Here's the drawing with two shaded views (mm, measured from the low corner). I have some questions. A direction names the side the tool comes from. Coordinates: 2 decimals unless noted, no trailing zeros. Order: outer loops, then holes, each group sorted by start corner. A loop starts at its lowest first (then second) coordinate and runs counter-clockwise, first axis right, second up. Notation, with made-up numbers: (-4.5, -9.5) -> (18.5, -9.5) arc R18 ccw to (18.5, 21.5) -> close; hole circle Ø7 at (59.5, -12.75). An arc over 180 degrees is marked (long way). Answer in a Markdown table with one row per item. Add a question column.
1. Imagine slicing it at D-D on z = 6. Write out the boundary of the cut face in (x, y).
2. On a 3-axis mill with a long thin cutter (end or side, diameter ignored), from which of +Z, -Z, +X, -X, +Y, -Y can I reach the whole of each face in a straight line? I mean the marked faces 1, 2 and 3. Say none if no direction works.
3. Will these pins go through, and if not, where does the flat tip stop? pin 1 (5 mm diameter, centred on y = 4.5, z = 12.5, fed in from -X); pin 2 (10 mm diameter, centred on y = 11, z = 10.5, fed in from +X).
4. Imagine slicing it at A-A on y = 10. Write out the boundary of the cut face in (x, z), plus the area to 3 significant figures.
5. Imagine slicing it at B-B on z = 22. Write out the boundary of the cut face in (x, y).
6. If I drill on line 1 along X through (y, z) = (3.5, 27.25); line 2 along Z through (x, y) = (2.5, 13.25), over which ranges is the centre line in solid material (lowest first)? Write a range as [from, to].
7. Imagine slicing it at C-C on x = 1.5. Write out the boundary of the cut face in (y, z), plus the area to 3 significant figures.
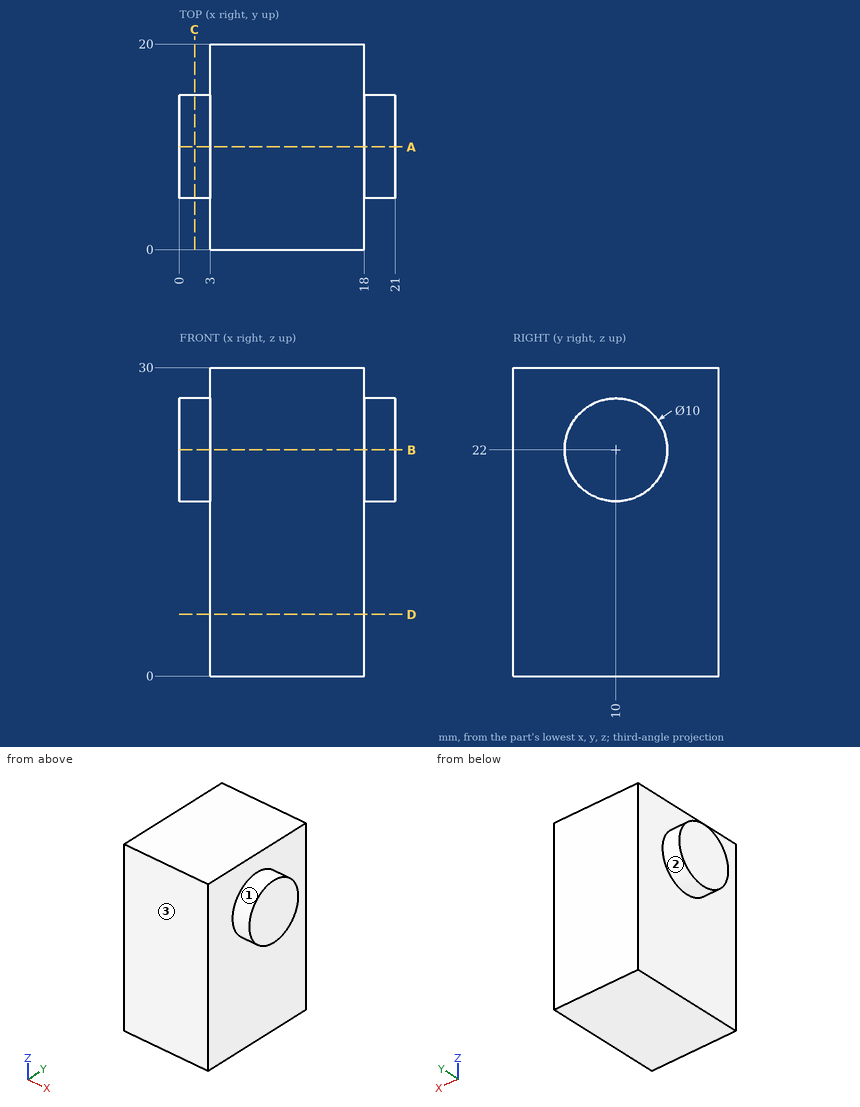
Answers follow:
| question | item | result |
|---|---|---|
| 1 | outline | (3, 0) -> (18, 0) -> (18, 20) -> (3, 20) -> close |
| 2 | face 1 | +X |
| 2 | face 2 | -X |
| 2 | face 3 | +Z, -Z, +X, -X, -Y |
| 3 | pin 1 | stops at x = 3 |
| 3 | pin 2 | stops at x = 18 |
| 4 | outline | (0, 17) -> (3, 17) -> (3, 0) -> (18, 0) -> (18, 17) -> (21, 17) -> (21, 27) -> (18, 27) -> (18, 30) -> (3, 30) -> (3, 27) -> (0, 27) -> close |
| 4 | area | 510 mm² |
| 5 | outline | (0, 5) -> (3, 5) -> (3, 0) -> (18, 0) -> (18, 5) -> (21, 5) -> (21, 15) -> (18, 15) -> (18, 20) -> (3, 20) -> (3, 15) -> (0, 15) -> close |
| 6 | line 1 | x = [3, 18] |
| 6 | line 2 | z = [18.2, 25.8] |
| 7 | outline | circle Ø10 at (10, 22) |
| 7 | area | 78.5 mm² |
